The drawing under review shows one solid part. Ordinate dimensions are in mm from its lowest x, y, z. A direction names the side the tool comes from. Give positions to 0.01 mm unless a question says otherwise; leave off trailing zeros. Order: outer loops, then holes, each group sorted by start corner. A loop starts at its lowest first (then second) coordinate and runs counter-clockwise, first axis right, second up. Notation, with made-up numbers: (55.5, 61.25) -> (73.5, 61.25) arc R17 ccw to (73.5, 81.25) -> close; hole circle Ø2 at (37.25, -4). An arc over 180 degrees is marked (long way). Return JSON: item names as keys, results as strings. Group by question number.
1) Insertion check: P1, Ø1.9, axis at x = 60.5, y = 2.5, coming from the +Z side. The pin has a flat end and moves straight along its axis. Give the tip position at first contact, or say it passes through.
2) For the marked faces 5 and 6, list the 3-axis set-ups (+Z, -Z, +X, -X, +Y, -Y) from which the entire face can be reached by the end or side of a thin tool; tool diameter is ignored.
3) The part is to be moulded in two halves that separate along Y. For the marked faces 1, 2, 3 and 4, say which applies: released by +Y, released by -Y, zero draft, split by the parting line, or undercut.
4) To check wall thickness, follow line 1 along Y through (x, z) = (24.5, 25); line 2 along X through (y, z) = (74.5, 25); line 3 along X through (y, z) = (81, 32.5) (1 decimal). State the ranges of each line that lie inside material, in increasing order.
5) Add section D-D (z = 13.5). Give the boundary of the cut face in (x, y) (1 decimal), then the cut area to 3 significant figures.
6) Add section B-B (z = 32.5). Give the boundary of the cut face in (x, y) (1 decimal).
7) Add section C-C (x = 74). Give the boundary of the cut face in (y, z).
8) Add section A-A (y = 66). Give the boundary of the cut face in (x, z).
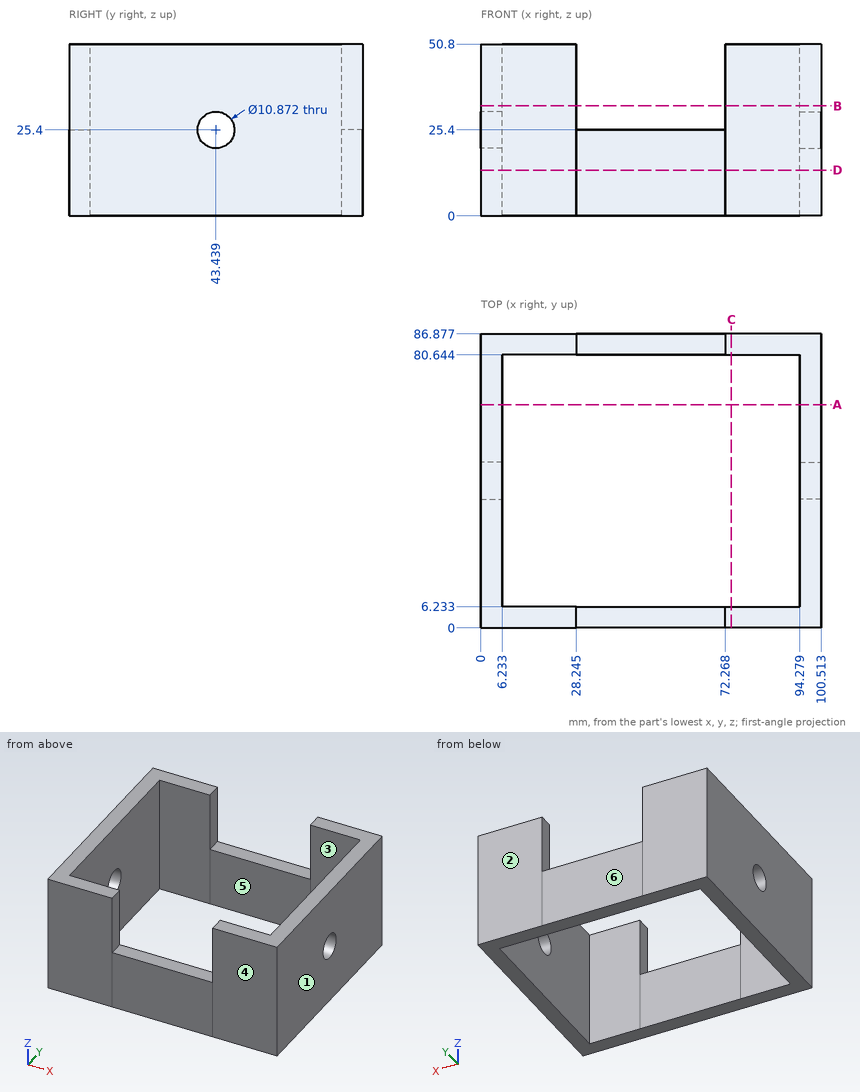
Evaluation:
{
 "1": {"P1": "z = 25.4"},
 "2": {"face 5": "+Z, -Z", "face 6": "+Z, -Z, +X, -X, +Y"},
 "3": {"face 1": "zero draft", "face 2": "released by +Y", "face 3": "undercut", "face 4": "released by -Y"},
 "4": {"line 1": "0 to 6.23, 80.64 to 86.88", "line 2": "0 to 6.23, 94.28 to 100.51", "line 3": "0 to 28.2, 72.3 to 100.5"},
 "5": {"outline": "(0, 0) -> (100.5, 0) -> (100.5, 86.9) -> (0, 86.9) -> close; hole (6.2, 6.2) -> (94.3, 6.2) -> (94.3, 80.6) -> (6.2, 80.6) -> close", "area": "2,180 mm^2"},
 "6": {"outline": "(0, 0) -> (28.2, 0) -> (28.2, 6.2) -> (6.2, 6.2) -> (6.2, 80.6) -> (28.2, 80.6) -> (28.2, 86.9) -> (0, 86.9) -> close; (72.3, 0) -> (100.5, 0) -> (100.5, 86.9) -> (72.3, 86.9) -> (72.3, 80.6) -> (94.3, 80.6) -> (94.3, 6.2) -> (72.3, 6.2) -> close"},
 "7": {"outline": "(0, 0) -> (6.23, 0) -> (6.23, 50.8) -> (0, 50.8) -> close; (80.64, 0) -> (86.88, 0) -> (86.88, 50.8) -> (80.64, 50.8) -> close"},
 "8": {"outline": "(0, 0) -> (6.23, 0) -> (6.23, 50.8) -> (0, 50.8) -> close; (94.28, 0) -> (100.51, 0) -> (100.51, 50.8) -> (94.28, 50.8) -> close"}
}
